Autodesk Fusion 360 part; units mm, degrees
sketch "Sketch1" plane through (0, 0, 0) normal (0, 0, 1) x (1, 0, 0)
  line L0 (0, 0) -> (150, 0)
  line L1 (150, 0) -> (150, 100)
  line L2 (150, 100) -> (0, 100)
  line L3 (0, 100) -> (0, 0)
  dimension "d1" = 100
  dimension "d2" = 150
extrude "Extrude1" add sketch "Sketch1" along normal blind 10
sketch "Sketch2" plane through (0, 0, 10) normal (0, 0, 1) x (-1, 0, 0)
  line L0 (0, -100) -> (0, 0)
  line L1 (0, 0) -> (-150, 0)
  line L2 (-150, 0) -> (-150, -100)
  line L3 (-150, -100) -> (0, -100)
  line L4 (-38.5, -75) -> (-61.5, -75)
  line L5 (-61.5, -75) -> (-61.5, -67)
  line L6 (-61.5, -67) -> (-38.5, -67)
  line L7 (-38.5, -67) -> (-38.5, -75)
  line L8 (-111.5, -75) -> (-88.5, -75)
  line L9 (-88.5, -75) -> (-88.5, -67)
  line L10 (-88.5, -67) -> (-111.5, -67)
  line L11 (-111.5, -67) -> (-111.5, -75)
  dimension "d5" = 8
  dimension "d6" = 23
  dimension "d7" = 38.5
  dimension "d8" = 23
  dimension "d9" = 8
  dimension "d10" = 38.5
  dimension "d11" = 25
  dimension "d12" = 25
sketch "Sketch3" plane through (0, 0, 10) normal (0, 0, 1) x (-1, 0, 0)
  line L0 (-38.5, -25) -> (-61.5, -25)
  line L1 (-61.5, -25) -> (-61.5, -33)
  line L2 (-61.5, -33) -> (-38.5, -33)
  line L3 (-38.5, -33) -> (-38.5, -25)
  line L4 (0, -100) -> (0, 0)
  line L5 (0, 0) -> (-150, 0)
  line L6 (-111.5, -25) -> (-88.5, -25)
  line L7 (-88.5, -25) -> (-88.5, -33)
  line L8 (-88.5, -33) -> (-111.5, -33)
  line L9 (-111.5, -33) -> (-111.5, -25)
  line L10 (-150, 0) -> (-150, -100)
  dimension "d13" = 8
  dimension "d14" = 23
  dimension "d15" = 38.5
  dimension "d16" = 25
  dimension "d17" = 8
  dimension "d18" = 23
  dimension "d19" = 38.5
  dimension "d20" = 25
extrude "Extrude2" cut sketch "Sketch3" against normal blind 7
extrude "Extrude3" cut sketch "Sketch2" against normal blind 7 contours L4 L5 L6 L7 | L8 L9 L10 L11
sketch "Sketch4" plane through (0, 0, 3) normal (0, 0, 1) x (-1, 0, 0)
  line L0 (-38.5, -67) -> (-61.5, -67)
  line L1 (-61.5, -67) -> (-61.5, -75)
  line L2 (-61.5, -75) -> (-38.5, -75)
  line L3 (-38.5, -75) -> (-38.5, -67)
  line L4 (-38.5, -25) -> (-38.5, -33)
  circle A0 centre (-50, -29) radius 4
  line L5 (-61.5, -25) -> (-38.5, -25)
  line L6 (-61.5, -33) -> (-61.5, -25)
  circle A1 centre (-50, -71) radius 4
  circle A2 centre (-100, -71) radius 4
  line L7 (-111.5, -75) -> (-111.5, -67)
  line L8 (-88.5, -75) -> (-111.5, -75)
  circle A3 centre (-100, -29) radius 4
  line L9 (-111.5, -33) -> (-111.5, -25)
  line L10 (-88.5, -33) -> (-111.5, -33)
  dimension "d27" = 8
  dimension "d28" = 4
  dimension "d29" = 11.5
  dimension "d30" = 8
  dimension "d31" = 11.5
  dimension "d32" = 4
  dimension "d33" = 8
  dimension "d34" = 11.5
  dimension "d35" = 4
  dimension "d36" = 8
  dimension "d37" = 11.5
  dimension "d38" = 4
extrude "Extrude4" add sketch "Sketch4" along normal blind 7 contours A1 | A0 | A2 | A3
sketch "Sketch5" plane through (0, 0, 0) normal (0, 0, 1) x (1, 0, 0)
sketch "Sketch6" plane through (0, 0, 10) normal (0, 0, 1) x (-1, 0, 0)
  line L0 (-61.5, -75) -> (-61.5, -67)
  line L1 (-61.5, -67) -> (-50, -67)
  line L2 (-50, -67) -> (-38.5, -67)
  line L3 (-38.5, -67) -> (-38.5, -75)
  line L4 (-38.5, -75) -> (-50, -75)
  line L5 (-50, -75) -> (-61.5, -75)
  line L6 (-88.5, -75) -> (-100, -75)
  line L7 (-100, -75) -> (-111.5, -75)
  line L8 (-111.5, -75) -> (-111.5, -67)
  line L9 (-111.5, -67) -> (-100, -67)
  line L10 (-100, -67) -> (-88.5, -67)
  line L11 (-88.5, -67) -> (-88.5, -75)
  line L12 (-88.5, -25) -> (-88.5, -33)
  line L13 (-88.5, -33) -> (-100, -33)
  line L14 (-100, -33) -> (-111.5, -33)
  line L15 (-111.5, -33) -> (-111.5, -25)
  line L16 (-111.5, -25) -> (-100, -25)
  line L17 (-100, -25) -> (-88.5, -25)
  line L18 (-61.5, -25) -> (-50, -25)
  line L19 (-50, -25) -> (-38.5, -25)
  line L20 (-38.5, -25) -> (-38.5, -33)
  line L21 (-38.5, -33) -> (-50, -33)
  line L22 (-50, -33) -> (-61.5, -33)
  line L23 (-61.5, -33) -> (-61.5, -25)
  line L24 (0, -100) -> (0, 0)
  line L25 (0, 0) -> (-150, 0)
  line L26 (-150, 0) -> (-150, -100)
  line L27 (-150, -100) -> (0, -100)
  line L28 (0, -100) -> (-5, -100)
  line L29 (-5, -100) -> (-5, 0)
  line L30 (-5, 0) -> (0, 0)
  line L31 (0, 0) -> (0, -100)
  line L32 (-150, -100) -> (-145, -100)
  line L33 (-145, -100) -> (-145, 0)
  line L34 (-145, 0) -> (-150, 0)
  line L35 (-150, 0) -> (-150, -100)
  dimension "d42" = 5
  dimension "d43" = 100
  dimension "d44" = 5
extrude "Extrude5" add sketch "Sketch6" along normal blind 15 contours L24 L25 L27 L28 L29 L30 L31 | L25 L26 L27 L32 L33 L34 L35
sketch "Sketch7" plane through (0, 0, 10) normal (0, 0, 1) x (-1, 0, 0)
  line L0 (-145, 0) -> (-145, -100)
  line L1 (-145, -100) -> (-5, -100)
  line L2 (-5, -100) -> (-5, 0)
  line L3 (-5, 0) -> (-145, 0)
  line L4 (-61.5, -25) -> (-50, -25)
  line L5 (-50, -25) -> (-38.5, -25)
  line L6 (-38.5, -25) -> (-38.5, -33)
  line L7 (-38.5, -33) -> (-50, -33)
  line L8 (-50, -33) -> (-61.5, -33)
  line L9 (-61.5, -33) -> (-61.5, -25)
  line L10 (-88.5, -25) -> (-88.5, -33)
  line L11 (-88.5, -33) -> (-100, -33)
  line L12 (-100, -33) -> (-111.5, -33)
  line L13 (-111.5, -33) -> (-111.5, -25)
  line L14 (-111.5, -25) -> (-100, -25)
  line L15 (-100, -25) -> (-88.5, -25)
  line L16 (-88.5, -75) -> (-100, -75)
  line L17 (-100, -75) -> (-111.5, -75)
  line L18 (-111.5, -75) -> (-111.5, -67)
  line L19 (-111.5, -67) -> (-100, -67)
  line L20 (-100, -67) -> (-88.5, -67)
  line L21 (-88.5, -67) -> (-88.5, -75)
  line L22 (-61.5, -75) -> (-61.5, -67)
  line L23 (-61.5, -67) -> (-50, -67)
  line L24 (-50, -67) -> (-38.5, -67)
  line L25 (-38.5, -67) -> (-38.5, -75)
  line L26 (-38.5, -75) -> (-50, -75)
  line L27 (-50, -75) -> (-61.5, -75)
  circle A0 centre (-140, -10) radius 2
  circle A1 centre (-10, -10) radius 2
  circle A2 centre (-10, -90) radius 2
  circle A3 centre (-140, -90) radius 2
  line L28 (0, -100) -> (0, 0)
  line L29 (-150, 0) -> (-150, -100)
  dimension "d47" = 4
  dimension "d48" = 4
  dimension "d49" = 4
  dimension "d50" = 4
  dimension "d51" = 10
  dimension "d52" = 10
  dimension "d53" = 10
  dimension "d54" = 10
  dimension "d55" = 10
  dimension "d56" = 10
  dimension "d57" = 10
  dimension "d58" = 10
extrude "Extrude6" cut sketch "Sketch7" against normal blind 10 contours A0 | A1 | A2 | A3
Can you work these out from the model? Positions are in its coordinate system, mm. A direction names the side the tool comes from. Give positions to 0.01 mm unless a question says otherwise; leave off trailing zeros. Order: outer loops, then holes, each group sorted by start corner. A loop starts at its lowest first (then second) coordinate and runs counter-clockwise, first axis right, second up. Notation, with made-up numbers: M 33,3.25 L 74,3.25 A35 cw 74,36.25 Z; hole C -26,3.25 d6. An arc over 180 degrees is marked long. Write item = value, one per line. Start each with the question number.
Q1. Will this pin go through, and if not, where does the flat tip stop? pin 1 Ø9 at (x, y) = (93.5, 71.5) entering from +Z.
Q2. Suppose I cut it at A-A (x = 140). Write out the boundary of the cut face in (y, z), plus the area to 3 significant figures.
Q3. Suppose I cut it at D-D (y = 29). Write out the boundary of the cut face in (x, z).
Q4. I need wall thicknesses on probe 1 along Y at (x, z) = (10, 7.75); probe 2 along X at (y, z) = (10, 4.25); probe 3 along X at (y, z) = (31, 11.75). Which ranges of each line are inside material? Lowest first, please. Write a range as [from, to].
Q5. For faces 3 (the flat face through (57, 29, 3)), 4 (the cylindrical face through (141.474, 88.648, 5.07)), 5 (the flat face through (100, 71, 10)), which set-ups out of +Z, -Z, +X, -X, +Y, -Y let a thin tool reach every point of the face, with its end or its side?
Q6. Suppose I cut it at B-B (z = 17). Write out the boundary of the cut face in (x, y), plus the area to 3 significant figures.
Q7. Suppose I cut it at C-C (y = 90). Write out the boundary of the cut face in (x, z).
Q8. We'd pull the mould along Y, two halves only. Please class faces 1 (the flat face through (148, 49, 25)), 2 (the cylindrical face through (142, 10, 5)): pulls with the +Y half, pulls with the -Y half, needs draft (parallel to the pull), parting line crosses it, or undercut.
Check result:
q1.pin_1 = 10
q2.outline = M 0,0 L 8,0 L 8,10 L 0,10 Z; M 12,0 L 88,0 L 88,10 L 12,10 Z; M 92,0 L 100,0 L 100,10 L 92,10 Z
q2.area = 920 mm2
q3.outline = M 0,0 L 150,0 L 150,25 L 145,25 L 145,10 L 111.5,10 L 111.5,3 L 104,3 L 104,10 L 96,10 L 96,3 L 88.5,3 L 88.5,10 L 61.5,10 L 61.5,3 L 54,3 L 54,10 L 46,10 L 46,3 L 38.5,3 L 38.5,10 L 5,10 L 5,25 L 0,25 Z
q4.probe_1 = [0, 8], [12, 88], [92, 100]
q4.probe_2 = [0, 8], [12, 138], [142, 150]
q4.probe_3 = [0, 5], [145, 150]
q5.face_3 = +Z
q5.face_4 = +Z, -Z
q5.face_5 = +Z, +Y, -Y
q6.outline = M 0,0 L 5,0 L 5,100 L 0,100 Z; M 145,0 L 150,0 L 150,100 L 145,100 Z
q6.area = 1,000 mm2
q7.outline = M 0,0 L 8,0 L 8,10 L 5,10 L 5,25 L 0,25 Z; M 12,0 L 138,0 L 138,10 L 12,10 Z; M 142,0 L 150,0 L 150,25 L 145,25 L 145,10 L 142,10 Z
q8.face_1 = needs draft
q8.face_2 = undercut
